Model file for the job. Use its own axes, mm. Face numbers are marked on the shaded views. A direction names the side the tool comes from. Round coordinates to 2 decimals unless told otherwise and drop trailing zeros. Order: outer loops, then holes, each group sorted by start corner. A loop starts at its lowest first (then second) coordinate and runs counter-clockwise, first axis right, second up. Notation, with made-up numbers: (17, 62) -> (61, 62) arc R13 cw to (61, 70) -> close; hole circle Ø2 at (-39.75, -39). An arc over 180 degrees is marked (long way). Answer as CSV lines item,"result".
```python
from build123d import *

# Parameters (mm, degrees)
SKETCH1_W           = 101.4
SKETCH1_H           = 56
SKETCH1_R           = 0.8
BOSS_EXTRUDE1_DEPTH = 1.6
SKETCH2_W           = 25
SKETCH2_H           = 19.6
SKETCH2_W_2         = 24.65
SKETCH2_H_2         = 20.5
BOSS_EXTRUDE2_DEPTH = 25
SKETCH3_R           = 1.5
CUT_EXTRUDE1_DEPTH  = 121.04903165
SKETCH4_R           = 10.9
BOSS_EXTRUDE3_DEPTH = 3
SKETCH5_W           = 9
SKETCH5_H           = 14.1
SKETCH5_W_2         = 24.4
SKETCH5_H_2         = 9
BOSS_EXTRUDE4_DEPTH = 11


with BuildPart() as part:
    # Sketch1 → Boss-Extrude1 (new body)
    with BuildSketch(Plane(origin=(0, 0, 0), x_dir=(1, 0, 0), z_dir=(0, 1, 0))):
        with Locations((50.7, 28)):
            Rectangle(SKETCH1_W, SKETCH1_H)
        with Locations(Location((2.7, 54, 0), (0, 0, 270))):
            Circle(SKETCH1_R, mode=Mode.SUBTRACT)
        with Locations(Location((2.7, 2.9, 0), (0, 0, 270))):
            Circle(SKETCH1_R, mode=Mode.SUBTRACT)
        with Locations(Location((99, 2.9, 0), (0, 0, 270))):
            Circle(SKETCH1_R, mode=Mode.SUBTRACT)
        with Locations(Location((99, 54, 0), (0, 0, 270))):
            Circle(SKETCH1_R, mode=Mode.SUBTRACT)
    extrude(amount=BOSS_EXTRUDE1_DEPTH)

    # Sketch2 → Boss-Extrude2 (add)
    with BuildSketch(Plane(origin=(0, 1.6, 0), x_dir=(1, 0, 0), z_dir=(0, 1, 0))):
        with Locations((18.7, 48.2)):
            Rectangle(SKETCH2_W, SKETCH2_H)
        with Locations((44.675, 48.25)):
            Rectangle(SKETCH2_W_2, SKETCH2_H_2)
    extrude(amount=BOSS_EXTRUDE2_DEPTH)

    # Sketch3 → Cut-Extrude1 (cut, through all)
    with BuildSketch(Plane(origin=(0, 0, -58.5), x_dir=(-1, 0, 0), z_dir=(0, 0, -1))):
        with Locations((-54.2, 23.45)):
            Circle(SKETCH3_R)
        with Locations((-34.2, 4.1)):
            Circle(SKETCH3_R)
        with Locations((-28.2, 23.45)):
            Circle(SKETCH3_R)
        with Locations((-8.2, 4.1)):
            Circle(SKETCH3_R)
    extrude(amount=-CUT_EXTRUDE1_DEPTH, mode=Mode.SUBTRACT)

    # Sketch4 → Boss-Extrude3 (add)
    with BuildSketch(Plane(origin=(0, 0, -58), x_dir=(-1, 0, 0), z_dir=(0, 0, -1))):
        with Locations(Location((-18.7, 13.9, 0), (0, 0, 180))):
            Circle(SKETCH4_R)
        with Locations(Location((-44.675, 13.9, 0), (0, 0, 180))):
            Circle(SKETCH4_R)
    extrude(amount=BOSS_EXTRUDE3_DEPTH)

    # Sketch5 → Boss-Extrude4 (add)
    with BuildSketch(Plane(origin=(0, 1.6, 0), x_dir=(1, 0, 0), z_dir=(0, 1, 0))):
        with Locations((64.7, 52.35)):
            Rectangle(SKETCH5_W, SKETCH5_H)
        with Locations((83.8, 54.9)):
            Rectangle(SKETCH5_W_2, SKETCH5_H_2)
    extrude(amount=BOSS_EXTRUDE4_DEPTH)


solid = part.part
```
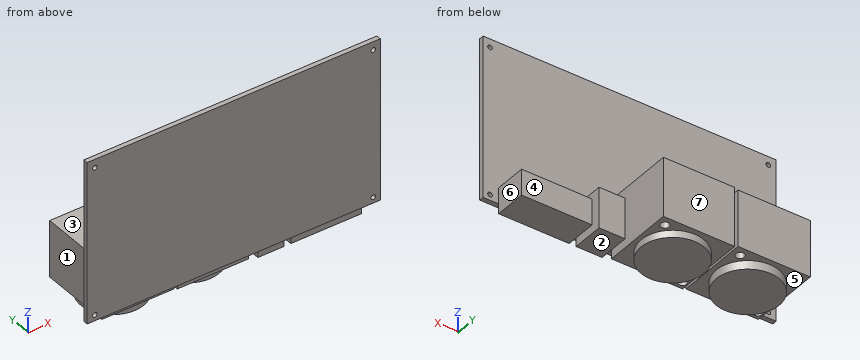
Q1. Saw through at C-C (y = 23.45). Write the cut outline in (x, z).
Checks:
outline,"(6.2, -58) -> (13.45, -58) -> (13.45, -61) -> (23.95, -61) -> (23.95, -58) -> (26.7, -58) -> (26.7, -38.4) -> (6.2, -38.4) -> close; (29.7, -58) -> (31.2, -58) -> (31.2, -38.4) -> (29.7, -38.4) -> close; (32.35, -58.5) -> (39.42, -58.5) -> (39.42, -61) -> (49.93, -61) -> (49.93, -58.5) -> (52.7, -58.5) -> (52.7, -38) -> (32.35, -38) -> close; (55.7, -58.5) -> (57, -58.5) -> (57, -38) -> (55.7, -38) -> close"
Q2. Mould opens along X. For the marked faces 5, 6 and 7 say: +X half, -X half, draft (parallel to the pull), parting line (faces both ways), or undercut.
Checks:
face 5,"undercut"
face 6,"+X half"
face 7,"draft"
Q3. Wall check: L1, parallel to X at y = 0.8, z = -54; L2, parallel to X at y = 21.5, z = -51; L3, parallel to Z at x = 99, y = 1.05. Give the ranges that are in metal, low to high. Write a range as [from, to].
Checks:
L1,"[0, 1.9], [3.5, 98.2], [99.8, 101.4]"
L2,"[6.2, 31.2], [32.35, 57]"
L3,"[-56, -54.8], [-53.2, -3.7], [-2.1, 0]"
Q4. Saw through at B-B (x = 28.2). Write the cut outline in (y, z), plus the area to 3 significant figures.
Checks:
outline,"(0, -56) -> (1.6, -56) -> (1.6, -58) -> (8.56, -58) -> (8.56, -61) -> (19.24, -61) -> (19.24, -58) -> (21.95, -58) -> (21.95, -38.4) -> (1.6, -38.4) -> (1.6, 0) -> (0, 0) -> close; (24.95, -58) -> (26.6, -58) -> (26.6, -38.4) -> (24.95, -38.4) -> close"
area,"553 mm²"
Q5. Flat gauge pins, fed straight in: pin 1 (10 mm diameter, centred on y = 11, z = -36, fed in from +X); pin 2 (4.5 mm diameter, centred on x = 81, z = -55, fed in from +Y); pin 3 (6 mm diameter, centred on x = 14.5, y = 17.5, fed in from +Z). Where does each tip first touch, or does it go through?
Checks:
pin 1,"x = 57"
pin 2,"y = 12.6"
pin 3,"z = -38.4"
Q6. Saw through at A-A (z = -47.5). Write the cut outline in (x, y).
Checks:
outline,"(0, 0) -> (101.4, 0) -> (101.4, 1.6) -> (69.2, 1.6) -> (69.2, 12.6) -> (60.2, 12.6) -> (60.2, 1.6) -> (57, 1.6) -> (57, 26.6) -> (32.35, 26.6) -> (32.35, 1.6) -> (31.2, 1.6) -> (31.2, 26.6) -> (6.2, 26.6) -> (6.2, 1.6) -> (0, 1.6) -> close; hole circle Ø3 at (8.2, 4.1); hole circle Ø3 at (28.2, 23.45); hole circle Ø3 at (34.2, 4.1); hole circle Ø3 at (54.2, 23.45)"
Q7. Tool access for the marked faces 1, 2, 3 and 4: list every direction of +Z, -Z, +X, -X, +Y, -Y with a clear straight run to the whole face (end or side of a thin tool).
Checks:
face 1,"+Z, -Z, -X, +Y"
face 2,"-Z, +X, +Y, -Y"
face 3,"+Z, -X, +Y"
face 4,"+Z, -Z, +X, +Y"
Q8. Saw through at D-D (x = 89.5). Write the cut outline in (y, z), plus the area to 3 significant figures.
Checks:
outline,"(0, -56) -> (1.6, -56) -> (1.6, -59.4) -> (12.6, -59.4) -> (12.6, -50.4) -> (1.6, -50.4) -> (1.6, 0) -> (0, 0) -> close"
area,"189 mm²"
